The listing builds one solid part. Answer for the finished solid, in the listing's coordinates (mm). Face numbers are marked on the shaded views. Coordinates: 2 decimals unless noted, no trailing zeros. Order: outer loops, then holes, each group sorted by start corner. A loop starts at its lowest first (then second) coordinate and runs counter-clockwise, first axis right, second up. Notation, with made-up numbers: M -28.75,-25.75 L 0.25,-25.75 A8 cw 0.25,-17.75 Z; hole C 74.5,69 d6. An arc over 180 degrees is marked long. One line per item, written item: value. Start each with the question number.
Q1. Determine the mould class of the marked faces 1, 2, 3 and 4 for opening direction Z: pulls with the +Z half, pulls with the -Z half, needs draft (parallel to the pull), parting line crosses it, or undercut.
Q2. The part is cut by section A-A on z = 24. Give the vertices of the cut face in (x, y).
Q3. Straight lines are drawn through the part: line 1 along Z through (x, y) = (8.5, -16); line 2 along Y through (x, z) = (-4.5, 26). For each, find the intervals that lie inside material, in ascending order. Write a range as [from, to].
Q4. The part is cut by section D-D on x = -16. Give the vertices of the cut face in (y, z), then the cut area to 3 significant figures.
Q5. Each of these flat-tipped pins is pushed along its axis until it touches: pin 1 Ø3 at (x, z) = (10, 43.5) entering from +Y; pin 2 Ø5 at (x, y) = (10.84, 12.18) entering from -Z; pin 3 Ø3.5 at (x, y) = (10.84, -18.82) entering from +Z. Where does it stop, or does it pass through?
Q6. The part is cut by section C-C on x = -10. Give the vertices of the cut face in (y, z).
Q7. The part is cut by section B-B on y = -13. Give the vertices of the cut face in (x, z), then the cut area to 3 significant figures.
```python
from build123d import *

# Parameters (mm, degrees)
SKETCH1_W            = 42.3
SKETCH1_H            = 42.3
BOSS_EXTRUDE1_DEPTH  = 1
SKETCH3_R            = 0.5
CUT_EXTRUDE1_DEPTH   = 2
CHAMFER1_SIZE        = 2.5
SKETCH4_R            = 12
CUT_EXTRUDE2_DEPTH   = 2
SKETCH5_R            = 1.5
CUT_EXTRUDE3_DEPTH   = 2
SKETCH6_W            = 42.3
SKETCH6_H            = 1
BOSS_EXTRUDE2_DEPTH  = 3.21
SKETCH7_W            = 42.3
SKETCH7_H            = 5.71
BOSS_EXTRUDE3_DEPTH  = 1
SKETCH8_W            = 42.3
SKETCH8_H            = 1
BOSS_EXTRUDE4_DEPTH  = 0.35
SKETCH9_W            = 42.3
SKETCH9_H            = 1
BOSS_EXTRUDE5_DEPTH  = 48
SKETCH10_W           = 42.3
SKETCH10_H           = 1
BOSS_EXTRUDE6_DEPTH  = 2.56
SKETCH11_W           = 49
SKETCH11_H           = 3.56
BOSS_EXTRUDE7_DEPTH  = 1
SKETCH12_W           = 5
SKETCH12_H           = 1
BOSS_EXTRUDE8_DEPTH  = 5
SKETCH13_W           = 49
SKETCH13_H           = 3.56
BOSS_EXTRUDE9_DEPTH  = 1
SKETCH14_W           = 5
SKETCH14_H           = 5
BOSS_EXTRUDE10_DEPTH = 3.56
SKETCH15_W           = 5
SKETCH15_H           = 2.56
CUT_EXTRUDE4_DEPTH   = 5
SKETCH16_R           = 1
CUT_EXTRUDE5_DEPTH   = 5
SKETCH17_W           = 5
SKETCH17_H           = 5
SKETCH17_R           = 1
BOSS_EXTRUDE11_DEPTH = 2.56
CUT_EXTRUDE6_DEPTH   = 5
SKETCH20_W           = 5
SKETCH20_H           = 3.56
BOSS_EXTRUDE12_DEPTH = 1
SKETCH21_W           = 6
SKETCH21_H           = 3.56
BOSS_EXTRUDE13_DEPTH = 1
SKETCH22_W           = 6
SKETCH22_H           = 3.56
BOSS_EXTRUDE14_DEPTH = 1
SKETCH23_W           = 5
SKETCH23_H           = 5
BOSS_EXTRUDE15_DEPTH = 2.56
SKETCH24_W           = 5
SKETCH24_H           = 3.56
BOSS_EXTRUDE16_DEPTH = 1
SKETCH25_W           = 5
SKETCH25_H           = 3.56
BOSS_EXTRUDE17_DEPTH = 1
SKETCH26_W           = 7
SKETCH26_H           = 3.56
BOSS_EXTRUDE18_DEPTH = 1
CUT_EXTRUDE7_DEPTH   = 21
SKETCH31_W           = 6
SKETCH31_H           = 7
CUT_EXTRUDE8_DEPTH   = 4.56
SKETCH32_W           = 6
SKETCH32_H           = 7
BOSS_EXTRUDE19_DEPTH = 2.56
BOSS_EXTRUDE20_START = -2.56
SKETCH34_W           = 6
SKETCH34_H           = 7
BOSS_EXTRUDE20_DEPTH = 2.56
SKETCH35_W           = 6
SKETCH35_H           = 7
CUT_EXTRUDE9_DEPTH   = 46.86


with BuildPart() as part:
    # Sketch1 → Boss-Extrude1 (new body)
    with BuildSketch(Plane.XY):
        with Locations((-4.664501511, -3.32265861)):
            Rectangle(SKETCH1_W, SKETCH1_H)
    extrude(amount=BOSS_EXTRUDE1_DEPTH)

    # Sketch3 → Cut-Extrude1 (cut, through all)
    with BuildSketch(Plane.XY.offset(1)):
        with Locations((-20.164501511, -18.82265861)):
            Circle(SKETCH3_R)
        with Locations((10.835498489, -18.82265861)):
            Circle(SKETCH3_R)
        with Locations((10.835498489, 12.17734139)):
            Circle(SKETCH3_R)
        with Locations((-20.164501511, 12.17734139)):
            Circle(SKETCH3_R)
    extrude(amount=-CUT_EXTRUDE1_DEPTH, mode=Mode.SUBTRACT)

    # Chamfer1
    chamfer1_edges = [part.edges().sort_by_distance(p)[0] for p in [
        (-25.814501511, 17.82734139, 0.5),
        (16.485498489, 17.82734139, 0.5),
        (16.485498489, -24.47265861, 0.5),
        (-25.814501511, -24.47265861, 0.5),
    ]]
    chamfer(chamfer1_edges, length=CHAMFER1_SIZE)

    # Sketch4 → Cut-Extrude2 (cut, through all)
    with BuildSketch(Plane.XY.offset(1)):
        with Locations((-4.664501511, -3.32265861)):
            Circle(SKETCH4_R)
    extrude(amount=-CUT_EXTRUDE2_DEPTH, mode=Mode.SUBTRACT)

    # Sketch5 → Cut-Extrude3 (cut, through all)
    with BuildSketch(Plane.XY.offset(1)):
        with Locations((-20.164501511, 12.17734139)):
            Circle(SKETCH5_R)
        with Locations((-20.164501511, -18.82265861)):
            Circle(SKETCH5_R)
        with Locations((10.835498489, -18.82265861)):
            Circle(SKETCH5_R)
        with Locations((10.835498489, 12.17734139)):
            Circle(SKETCH5_R)
    extrude(amount=-CUT_EXTRUDE3_DEPTH, mode=Mode.SUBTRACT)

    # Sketch6 → Boss-Extrude2 (add)
    with BuildSketch(Plane.XZ.offset(24.47265861)):
        with Locations((-4.664501511, 0.5)):
            Rectangle(SKETCH6_W, SKETCH6_H)
    extrude(amount=BOSS_EXTRUDE2_DEPTH)

    # Sketch7 → Boss-Extrude3 (add)
    with BuildSketch(Plane.XY.offset(1)):
        with Locations((-4.664501511, -24.82765861)):
            Rectangle(SKETCH7_W, SKETCH7_H)
    extrude(amount=-BOSS_EXTRUDE3_DEPTH)

    # Sketch8 → Boss-Extrude4 (add)
    with BuildSketch(Plane.XZ.offset(27.68265861)):
        with Locations((-4.664501511, 0.5)):
            Rectangle(SKETCH8_W, SKETCH8_H)
    extrude(amount=BOSS_EXTRUDE4_DEPTH)

    # Sketch9 → Boss-Extrude5 (add)
    with BuildSketch(Plane.XY.offset(1)):
        with Locations((-4.664501511, -24.97265861)):
            Rectangle(SKETCH9_W, SKETCH9_H)
    extrude(amount=BOSS_EXTRUDE5_DEPTH)

    # Sketch10 → Boss-Extrude6 (add)
    with BuildSketch(Plane.XZ.offset(25.47265861)):
        with Locations((-4.664501511, 48.5)):
            Rectangle(SKETCH10_W, SKETCH10_H)
    extrude(amount=BOSS_EXTRUDE6_DEPTH)

    # Sketch11 → Boss-Extrude7 (add)
    with BuildSketch(Plane.ZY.offset(25.814501511)):
        with Locations((24.5, -26.25265861)):
            Rectangle(SKETCH11_W, SKETCH11_H)
    extrude(amount=-BOSS_EXTRUDE7_DEPTH)

    # Sketch12 → Boss-Extrude8 (add)
    with BuildSketch(Plane.ZY.offset(25.814501511)):
        with Locations((24.5, -27.53265861)):
            Rectangle(SKETCH12_W, SKETCH12_H)
    extrude(amount=BOSS_EXTRUDE8_DEPTH)

    # Sketch13 → Boss-Extrude9 (add)
    with BuildSketch(Plane(origin=(16.485498489, 0, 0), x_dir=(0, 0, -1), z_dir=(1, 0, 0))):
        with Locations((-24.5, -26.25265861)):
            Rectangle(SKETCH13_W, SKETCH13_H)
    extrude(amount=-BOSS_EXTRUDE9_DEPTH)

    # Sketch14 → Boss-Extrude10 (add)
    with BuildSketch(Plane(origin=(0, -24.47265861, 0), x_dir=(1, 0, 0), z_dir=(0, 1, 0))):
        with Locations((18.985498489, -24.5)):
            Rectangle(SKETCH14_W, SKETCH14_H)
    extrude(amount=-BOSS_EXTRUDE10_DEPTH)

    # Sketch15 → Cut-Extrude4 (cut)
    with BuildSketch(Plane(origin=(21.485498489, 0, 0), x_dir=(0, 0, -1), z_dir=(1, 0, 0))):
        with Locations((-24.5, -25.75265861)):
            Rectangle(SKETCH15_W, SKETCH15_H)
    extrude(amount=-CUT_EXTRUDE4_DEPTH, mode=Mode.SUBTRACT)

    # Sketch16 → Cut-Extrude5 (cut)
    with BuildSketch(Plane(origin=(0, -27.03265861, 0), x_dir=(1, 0, 0), z_dir=(0, 1, 0))):
        with Locations((-28.314501511, -24.5)):
            Circle(SKETCH16_R)
        with Locations((18.985498489, -24.5)):
            Circle(SKETCH16_R)
    extrude(amount=-CUT_EXTRUDE5_DEPTH, mode=Mode.SUBTRACT)

    # Sketch17 → Boss-Extrude11 (add)
    with BuildSketch(Plane(origin=(0, -27.03265861, 0), x_dir=(1, 0, 0), z_dir=(0, 1, 0))):
        with Locations((-28.314501511, -24.5)):
            Rectangle(SKETCH17_W, SKETCH17_H)
        with Locations((-28.314501511, -24.5)):
            Circle(SKETCH17_R, mode=Mode.SUBTRACT)
    extrude(amount=BOSS_EXTRUDE11_DEPTH)

    # Sketch19 → Cut-Extrude6 (cut)
    with BuildSketch(Plane(origin=(0, -24.47265861, 0), x_dir=(1, 0, 0), z_dir=(0, 1, 0))):
        Polygon((-29.469202049, -26.5), (-27.159800972, -26.5), (-26.005100434, -24.5), (-27.159800972, -22.5), (-29.469202049, -22.5), (-30.623902587, -24.5), align=None)
    extrude(amount=-CUT_EXTRUDE6_DEPTH, mode=Mode.SUBTRACT)

    # Sketch20 → Boss-Extrude12 (add)
    with BuildSketch(Plane.ZY.offset(30.814501511)):
        with Locations((24.5, -26.25265861)):
            Rectangle(SKETCH20_W, SKETCH20_H)
    extrude(amount=BOSS_EXTRUDE12_DEPTH)

    # Sketch21 → Boss-Extrude13 (add)
    with BuildSketch(Plane.XY.offset(27)):
        with Locations((-28.814501511, -26.25265861)):
            Rectangle(SKETCH21_W, SKETCH21_H)
    extrude(amount=BOSS_EXTRUDE13_DEPTH)

    # Sketch22 → Boss-Extrude14 (add)
    with BuildSketch(Plane(origin=(0, 0, 22), x_dir=(-1, 0, 0), z_dir=(0, 0, -1))):
        with Locations((28.814501511, -26.25265861)):
            Rectangle(SKETCH22_W, SKETCH22_H)
    extrude(amount=BOSS_EXTRUDE14_DEPTH)

    # Sketch23 → Boss-Extrude15 (add)
    with BuildSketch(Plane(origin=(0, -27.03265861, 0), x_dir=(1, 0, 0), z_dir=(0, 1, 0))):
        with Locations((18.985498489, -24.5)):
            Rectangle(SKETCH23_W, SKETCH23_H)
    extrude(amount=BOSS_EXTRUDE15_DEPTH)

    # Sketch24 → Boss-Extrude16 (add)
    with BuildSketch(Plane.XY.offset(27)):
        with Locations((18.985498489, -26.25265861)):
            Rectangle(SKETCH24_W, SKETCH24_H)
    extrude(amount=BOSS_EXTRUDE16_DEPTH)

    # Sketch25 → Boss-Extrude17 (add)
    with BuildSketch(Plane(origin=(0, 0, 22), x_dir=(-1, 0, 0), z_dir=(0, 0, -1))):
        with Locations((-18.985498489, -26.25265861)):
            Rectangle(SKETCH25_W, SKETCH25_H)
    extrude(amount=BOSS_EXTRUDE17_DEPTH)

    # Sketch26 → Boss-Extrude18 (add)
    with BuildSketch(Plane(origin=(21.485498489, 0, 0), x_dir=(0, 0, -1), z_dir=(1, 0, 0))):
        with Locations((-24.5, -26.25265861)):
            Rectangle(SKETCH26_W, SKETCH26_H)
    extrude(amount=BOSS_EXTRUDE18_DEPTH)

    # Sketch29 → Cut-Extrude7 (cut)
    with BuildSketch(Plane(origin=(0, -24.47265861, 0), x_dir=(1, 0, 0), z_dir=(0, 1, 0))):
        Polygon((20.640199028, -26.5), (21.794899566, -24.5), (20.640199028, -22.5), (18.330797951, -22.5), (17.176097413, -24.5), (18.330797951, -26.5), align=None)
    extrude(amount=-CUT_EXTRUDE7_DEPTH, mode=Mode.SUBTRACT)

    # Sketch31 → Cut-Extrude8 (cut, through all)
    with BuildSketch(Plane(origin=(0, -24.47265861, 0), x_dir=(1, 0, 0), z_dir=(0, 1, 0))):
        with Locations((19.485498489, -24.5)):
            Rectangle(SKETCH31_W, SKETCH31_H)
    extrude(amount=-CUT_EXTRUDE8_DEPTH, mode=Mode.SUBTRACT)

    # Sketch32 → Boss-Extrude19 (add)
    with BuildSketch(Plane.XZ.offset(25.47265861)):
        with Locations((-21.814501511, 24.5)):
            Rectangle(SKETCH32_W, SKETCH32_H)
    extrude(amount=BOSS_EXTRUDE19_DEPTH)

    # Sketch34 → Boss-Extrude20 (add)
    with BuildSketch(Plane(origin=(0, -28.03265861, 0), x_dir=(-1, 0, 0), z_dir=(0, -1, 0)).offset(BOSS_EXTRUDE20_START)):
        with Locations((-12.485498489, -24.5)):
            Rectangle(SKETCH34_W, SKETCH34_H)
    extrude(amount=BOSS_EXTRUDE20_DEPTH)

    # Sketch35 → Cut-Extrude9 (cut, through all)
    with BuildSketch(Plane.XZ.offset(28.03265861)):
        with Locations((-28.814501511, 24.5)):
            Rectangle(SKETCH35_W, SKETCH35_H)
    extrude(amount=-CUT_EXTRUDE9_DEPTH, mode=Mode.SUBTRACT)


solid = part.part
```
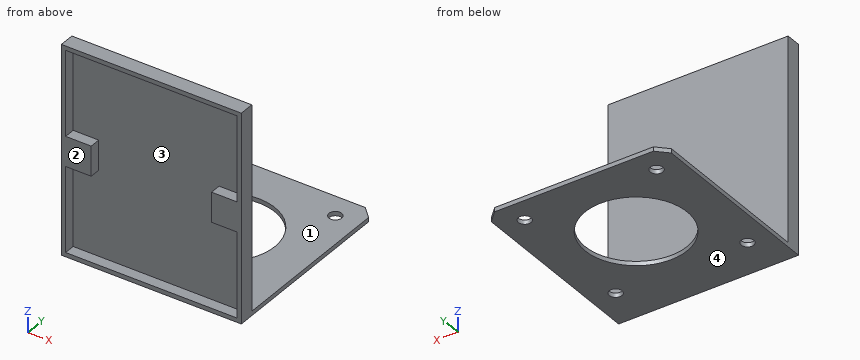
Output:
1. face 1: pulls with the +Z half
1. face 2: needs draft
1. face 3: undercut
1. face 4: pulls with the -Z half
2. outline: M -25.81,-28.03 L -18.81,-28.03 L -18.81,-25.47 L 9.49,-25.47 L 9.49,-28.03 L 16.49,-28.03 L 16.49,-24.47 L -25.81,-24.47 Z
3. line 1: z = [0, 1]
3. line 2: y = [-25.47, -24.47]
4. outline: M -28.03,0 L -7.26,0 L -7.26,1 L -24.47,1 L -24.47,49 L -28.03,49 L -28.03,48 L -25.47,48 L -25.47,1 L -28.03,1 Z; M 0.62,0 L 17.83,0 L 17.83,1 L 0.62,1 Z
4. area: 88.5 mm^2
5. pin 1: stops at y = -24.47
5. pin 2: stops at z = 0
5. pin 3: stops at z = 1
6. outline: M -28.03,0 L -14.07,0 L -14.07,1 L -24.47,1 L -24.47,49 L -28.03,49 L -28.03,48 L -25.47,48 L -25.47,1 L -28.03,1 Z; M 7.43,0 L 17.83,0 L 17.83,1 L 7.43,1 Z
7. outline: M -25.81,0 L -11.76,0 L -11.76,1 L -25.81,1 Z; M 2.43,0 L 16.49,0 L 16.49,1 L 2.43,1 Z
7. area: 28.1 mm^2
